Work out the finished part from the listing and answer in its coordinate system (mm). Give positions to 0.01 mm unless a question says otherwise; leave off trailing zeros. Loops run counter-clockwise (first coordinate to the right, second up) from the corner with the lowest first, then second, coordinate; pieces in that order, holes last. Notation, with made-up numbers: M -22,54.25 L 26,54.25 A34 ccw 26,89.25 Z; hole C 9,38 d5. An arc over 180 degrees is marked long. Write item = value, one per line. Start each with the question number.
1. Section A-A on y = -10 is taken. Determine the outline of the cut face in (x, z).
2. Consider L1, parallel to Z at x = -6.25, y = -3; L2, parallel to Y at x = -2.75, z = -0.35; L3, parallel to Z at x = -3, y = -28. Determine where each line is inside the solid, lowest interval first. Write a range as [from, to].
3. Flat-ended cylindrical pins translate along their axes: pin 1 Ø0.7 at (x, y) = (-2.975, -33) entering from +Z; pin 2 Ø2.5 at (x, y) = (-3.5, -32.5) entering from +Z; pin 3 Ø1.5 at (y, z) = (-12.5, 1) entering from +X; pin 4 Ø0.6 at (x, z) = (-3.5, -1) entering from +Y. Find the tip coordinate at first contact, or state that the pin passes through.
4. Section B-B on y = -20.5 is taken. Determine the outline of the cut face in (x, z), plus the area to 3 significant figures.
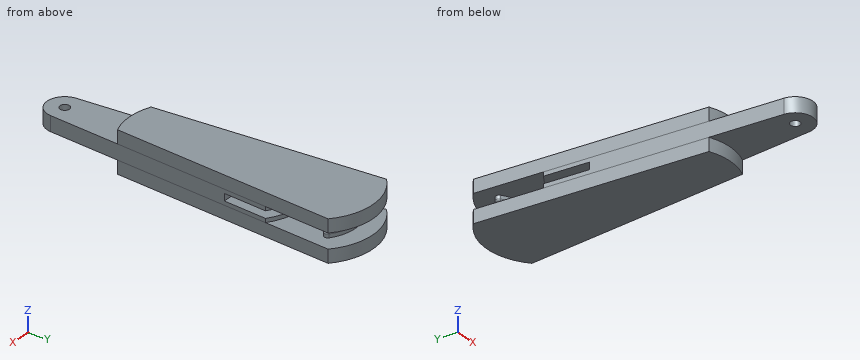
Autodesk Inventor part; units mm, degrees
ref_plane "Work Plane1" through (-4.9692, -33.1526, -0.85) normal (0, 0, -1) x (-1, 0, 0)
ref_plane "YZ Plane" through (0, 0, 0) normal (1, 0, 0) x (0, 1, 0)
ref_plane "XZ Plane" through (0, 0, 0) normal (0, 1, 0) x (-1, 0, 0)
sketch "Sketch1" plane through (0, 0, 0) normal (0, 0, 1) x (1, 0, 0)
  arc A0 (-0.1713, -0.9133) -> (-5.7787, -0.9133) centre (-2.975, -4.7604) ccw
  arc A1 (-5.7787, -1.5867) -> (-0.1713, -1.5867) centre (-2.975, 2.2604) ccw
  circle A2 centre (-5.5333, -1.25) radius 0.4167
  circle A3 centre (-0.4167, -1.25) radius 0.4167
  line L0 (-5.95, 0) -> (0, 0)
  line L1 (0, 0) -> (0, -2.5)
  line L2 (0, -2.5) -> (-5.95, -2.5)
  line L3 (-5.95, -2.5) -> (-5.95, 0)
  point P0 (-1.5, -3.25)
  dimension "d8" = 4.7604
  dimension "d11" = 0.8333
  dimension "d12" = 5.95
  dimension "d13" = 2.5
  dimension "d14" = 0.8333
  dimension "d22" = 4.7604
extrude "Extrusion1" add sketch "Sketch1" against normal blind 0.6 contours A3 A1 A2 A0 | A3 | A2
sketch "Sketch2" plane through (0, 0, 0) normal (0, 0, 1) x (1, 0, 0)
  arc A0 (-0.1713, -0.9133) -> (-5.7787, -0.9133) centre (-2.975, -4.7604) ccw
  arc A1 (1.575, 0.2396) -> (-7.525, 0.2396) centre (-2.975, -4.7604) ccw
  line L0 (-4.9692, -33.1526) -> (-7.525, 0.2396)
  line L1 (-0.9808, -33.1526) -> (1.575, 0.2396)
  circle A2 centre (-2.975, -33) radius 2
  arc A3 (-0.1713, -0.9133) -> (-5.7787, -0.9133) centre (-2.975, -4.7604) ccw
  line L2 (-11.9492, 2) -> (-1.5879, 2) construction
  point P0 (-7.5, -3.25)
  dimension "d15" = 33.4899
  dimension "d16" = 2
  dimension "d17" = 33.4899
  dimension "d19" = 4
  dimension "d20" = 9.1
  dimension "d21" = 35
extrude "Extrusion2" add sketch "Sketch2" along normal blind 1.5
sketch "Sketch4" plane through (0, 0, 0) normal (0, 0, -1) x (-1, 0, 0)
  arc A0 (7.525, 0.2396) -> (-1.575, 0.2396) centre (2.975, -4.7604) ccw
  line L0 (4.6338, -2.5) -> (0.9036, -2.5) construction
  line L1 (4.4698, -6) -> (1.0404, -6) construction
  arc A1 (0.1713, -1.5867) -> (5.7787, -1.5867) centre (2.975, 2.2604) ccw construction
  line L2 (7.525, 0.2396) -> (4.9692, -33.1526) construction
  line L3 (0.9808, -33.1526) -> (-1.575, 0.2396) construction
  arc A2 (6.9486, -7.2911) -> (-0.9986, -7.2911) centre (2.975, -12.7604) ccw
  line L4 (7.525, 0.2396) -> (4.9692, -33.1526) construction
  line L5 (0.9808, -33.1526) -> (-1.575, 0.2396) construction
  arc A3 (0.9808, -33.1526) -> (4.9692, -33.1526) centre (2.975, -33) ccw
  line L6 (6.9486, -7.2911) -> (4.9692, -33.1526)
  line L7 (0.9808, -33.1526) -> (-0.9986, -7.2911)
  point P0 (0, 0)
  dimension "d23" = 3.5
  dimension "d24" = 6.7604
  dimension "d25" = 6.7604
extrude "Extrusion4" add sketch "Sketch4" along normal blind 0.85
sketch "Sketch7" plane through (0, 0, -0.85) normal (0, 0, -1) x (-1, 0, 0)
  arc A0 (6.9486, -7.2911) -> (-0.9986, -7.2911) centre (2.975, -12.7604) ccw
  line L0 (-0.9986, -7.2911) -> (0.9808, -33.1526)
  arc A1 (0.9808, -33.1526) -> (4.9692, -33.1526) centre (2.975, -33) ccw
  line L1 (4.9692, -33.1526) -> (6.9486, -7.2911)
  line L2 (-0.6188, -12.2527) -> (6.5688, -12.2527)
  point P0 (0, 0)
extrude "Extrusion7" cut sketch "Sketch7" against normal blind 0.4 contours L1 L2 L0 A0
sketch "Sketch3" plane through (0, 0, 1.5) normal (0, 0, 1) x (1, 0, 0)
  arc A0 (-4.9692, -33.1526) -> (-0.9808, -33.1526) centre (-2.975, -33) ccw
  circle A1 centre (-2.975, -33) radius 0.55
  point P0 (0, 0)
  dimension "d5" = 1.1
extrude "Extrusion3" cut sketch "Sketch3" against normal through all
ref_plane "Work Plane1" through (-4.9692, -33.1526, -0.85) normal (0, 0, -1) x (-1, 0, 0)
mirror "Mirror1" about plane through (-2.975, -19.8303, -0.85) normal (0, 0, -1) of "Extrusion1", "Extrusion2", "Extrusion4", "Extrusion3", "Extrusion7"
sketch "Sketch8" plane through (-2.975, -4.7604, -3.2) normal (0, 0, -1) x (-1, 0, 0)
  circle A0 centre (0, -28.2396) radius 0.55
  arc A1 (-1.9942, -28.3923) -> (1.9942, -28.3923) centre (0, -28.2396) ccw
  line L0 (4.55, 5) -> (1.9942, -28.3923)
  arc A2 (4.55, 5) -> (-4.55, 5) centre (0, 0) ccw
  line L1 (-1.9942, -28.3923) -> (-4.55, 5)
  line L2 (-1.9942, -28.3923) -> (-4.55, 5)
  line L3 (4.55, 5) -> (1.9942, -28.3923)
  arc A3 (-2.6101, -20.3444) -> (2.6101, -20.3444) centre (0, -14.1082) ccw
  point P0 (-2.975, 4.7604)
  dimension "d37" = 6.7604
  dimension "d38" = 6.7604
extrude "Extrusion8" cut sketch "Sketch8" against normal blind 1.5 contours L1 A3 L0 A1
mirror "Mirror2" about plane through (-4.9692, -33.1526, -0.85) normal (0, 0, -1) of "Extrusion8"
fillet "Fillet1" radius 0.2 8 edges at (-2.975, 0, -0.6) (0, -1.25, -0.6) (-2.975, -2.5, -0.6) (-5.95, -1.25, -0.6) (-2.975, 0, -1.1) (0, -1.25, -1.1) (-2.975, -2.5, -1.1) (-5.95, -1.25, -1.1)
sketch "Sketch6" plane through (-2.975, -4.7604, -3.2) normal (0, 0, -1) x (-1, 0, 0)
  line L0 (-1.9942, -28.3923) -> (-4.55, 5)
  line L1 (4.55, 5) -> (1.9942, -28.3923)
  arc A0 (-2.5344, -21.3343) -> (2.5344, -21.3343) centre (0, -18.2396) ccw
  circle A1 centre (0, -28.2396) radius 0.55
  arc A2 (-1.9942, -28.3923) -> (1.9942, -28.3923) centre (0, -28.2396) ccw
  point P0 (-2.975, 4.7604)
  dimension "d31" = 4
  dimension "d32" = 10
equation "\"d11\" = 0.333333 * d13"
equation "\"d12\" = phheight"
equation "\"d13\" = phwidth"
equation "\"d14\" = d11"
equation "\"d22\" = d8"
equation "\"d16\" = phtosolid"
equation "\"d17\" = d15"
equation "\"d20\" = pheight"
equation "\"d24\" = d25"
equation "\"d37\" = d38"
equation "\"phtofree\" = 2.5"
equation "\"phtosolid\" = 2"
properties part number "poker"
Verdict:
q1.outline = M -6.74,-3.2 L 0.79,-3.2 L 0.79,-1.25 L -6.74,-1.25 Z; M -6.74,-0.45 L 0.79,-0.45 L 0.79,1.5 L -6.74,1.5 Z
q2.L1 = [-3.2, -1.7], [0, 1.5]
q2.L2 = [-34.99, -33.5], [-32.5, -6], [-2.49, -0.01]
q2.L3 = [-1.7, 0]
q3.pin_1 = through
q3.pin_2 = 0
q3.pin_3 = 0.66
q3.pin_4 = -0.02
q4.outline = M -5.94,-3.2 L -0.01,-3.2 L -0.01,1.5 L -5.94,1.5 L -5.94,0 Z
q4.area = 27.8 mm2
